Check sheet for the drawn part. Datum: minimum x, y, z corner. Units: mm. A direction names the side the tool comes from. Coordinates: 2 decimals unless noted, no trailing zeros. Order: outer loops, then holes, each group sorted by start corner. A loop starts at its lowest first (then second) coordinate and runs counter-clockwise, first axis right, second up. Notation, with made-up numbers: (7.5, 4.5) -> (11.5, 4.5) arc R24 cw to (11.5, 14.5) -> close; hole circle Ø8 at (-7, 53.5). An arc over 180 degrees is marked (long way). Write item = value, one per line. Start each with the question number.
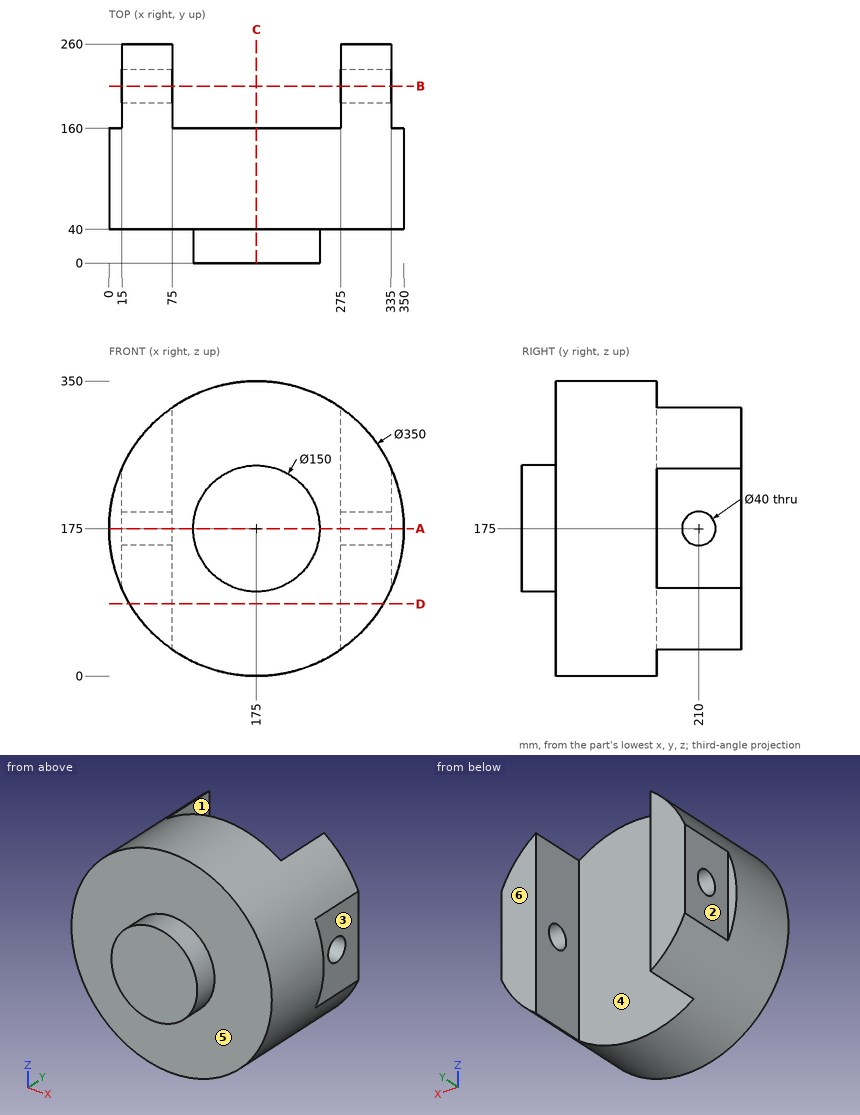
Item 1: Section check C-C (x = 175). Record the boundary of the cut face in (y, z).
Item 2: Section check B-B (y = 210). Record the boundary of the cut face in (x, z).
Item 3: Section check D-D (z = 85.5). Record the boundary of the cut face in (x, y), then the cut area to 3 significant figures.
Item 4: Mould release check, pull along X, two halves, no side actions. Record for the marked faces 1, 2 and 3: pulls with the +X half, pulls with the -X half, needs draft (parallel to the pull), parting line crosses it, or undercut.
Item 5: Gauge pin test, flat ends, axial feed: P1, Ø4, axis at x = 108.5, y = 75, coming from the -Z side; P2, Ø6, axis at x = 182, z = 215, coming from the +Y side; P3, Ø8, axis at x = 124, z = 297.5, coming from the -Y side. Record the tip position at first contact, or that the pin passes through.
Item 6: Thickness scan on line 1 (Y direction, x = 59.5, z = 175); line 2 (X direction, y = 160.5, z = 219.5); line 3 (Y direction, x = 212.5, z = 271). Record the ranges inside material, lowest first.
Item 7: Tool access check on the marked faces 4, 5 and 6. Record the directions out of +Z, -Z, +X, -X, +Y, -Y that give a thin tool (end or side, any length) a straight path to the whole face; none if there is none.
Item 8: Section check A-A (z = 175). Record the boundary of the cut face in (x, y).
Filled sheet:
q1.outline = (0, 100) -> (40, 100) -> (40, 0) -> (160, 0) -> (160, 350) -> (40, 350) -> (40, 250) -> (0, 250) -> close
q2.outline = (15, 104.11) arc R175 ccw to (75, 31.39) -> (75, 155) -> (15, 155) -> close; (15, 195) -> (75, 195) -> (75, 318.61) arc R175 ccw to (15, 245.89) -> close; (275, 31.39) arc R175 ccw to (335, 104.11) -> (335, 155) -> (275, 155) -> close; (275, 195) -> (335, 195) -> (335, 245.89) arc R175 ccw to (275, 318.61) -> close
q3.outline = (24.62, 40) -> (325.38, 40) -> (325.38, 260) -> (275, 260) -> (275, 160) -> (75, 160) -> (75, 260) -> (24.62, 260) -> close
q3.area = 46,200 mm^2
q4.face_1 = undercut
q4.face_2 = pulls with the -X half
q4.face_3 = pulls with the +X half
q5.P1 = 12.32
q5.P2 = 160
q5.P3 = 40
q6.line_1 = 40 to 190, 230 to 260
q6.line_2 = 15 to 75, 275 to 335
q6.line_3 = 40 to 160
q7.face_4 = +Z, -Z, +Y
q7.face_5 = -Y
q7.face_6 = +Z, -Z, +X, -X, +Y
q8.outline = (0, 40) -> (100, 40) -> (100, 0) -> (250, 0) -> (250, 40) -> (350, 40) -> (350, 160) -> (335, 160) -> (335, 190) -> (275, 190) -> (275, 160) -> (75, 160) -> (75, 190) -> (15, 190) -> (15, 160) -> (0, 160) -> close; (15, 230) -> (75, 230) -> (75, 260) -> (15, 260) -> close; (275, 230) -> (335, 230) -> (335, 260) -> (275, 260) -> close
